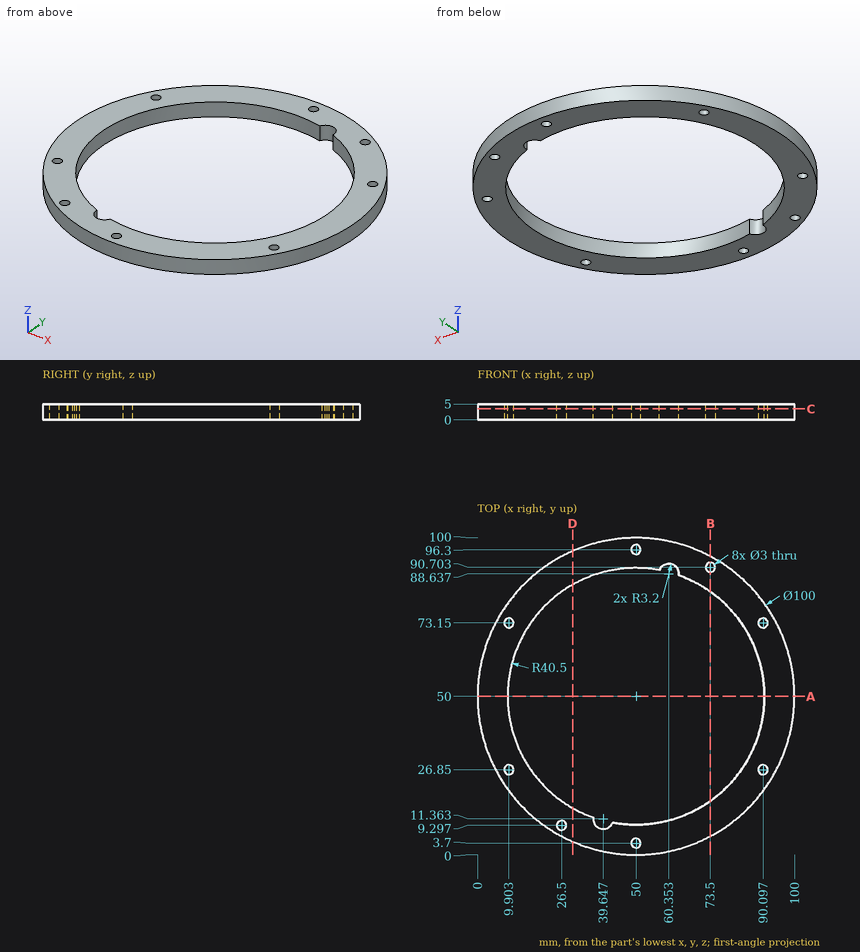
Can you work these out from the drawing? Everything is in mm from the part's minimum corner. Give positions to 0.01 mm unless a question says otherwise; leave off trailing zeros. Order: outer loops, then holes, each group sorted by start corner. A loop starts at its lowest first (then second) coordinate and runs counter-clockwise, first axis right, second up. Notation, with made-up numbers: M -8.5,88.5 L 25.5,88.5 A11 cw 25.5,107.5 Z; hole C 81,82.5 d3. An arc over 180 degrees is marked long. Use a Markdown table: item, result. Add a question column.
Item 1: Suppose I cut it at B-B (x = 73.5). List the corners of the cut face in (y, z) for me (1 decimal).
Item 2: Suppose I cut it at A-A (y = 50). List the corners of the cut face in (x, z) for me, then the cut area to 3 significant figures.
Item 3: If I drill on L1, parallel to Y at x = 50, z = 3.05; L2, parallel to Y at x = 50.5, z = 3.7 (1 decimal); L3, parallel to X at y = 8.5, z = 1.3 (1 decimal), over which ranges is the centre line in solid material (lowest first)? Write a range as [from, to].
Item 4: Suppose I cut it at D-D (x = 30). List the corners of the cut face in (y, z) for me, then the cut area to 3 significant figures.
Item 5: Will these pins go through, and if not, where does the flat tip stop? pin 1 (2.5 mm diameter, centred on x = 50, y = 3.7, fed in from +Z); pin 2 (1.5 mm diameter, centred on x = 23, z = 4.5, fed in from +Y) (1 decimal); pin 3 (1 mm diameter, centred on y = 30.5, z = 3, fed in from +X).
Item 6: Suppose I cut it at C-C (z = 3.5). Count the separate pieces of the cut face and the enclosed holes in it, then the cut area to 3 significant figures.
Answer sheet:
| question | item | result |
|---|---|---|
| 1 | outline | M 5.9,0 L 17,0 L 17,5 L 5.9,5 Z; M 83,0 L 89.2,0 L 89.2,5 L 83,5 Z; M 92.2,0 L 94.1,0 L 94.1,5 L 92.2,5 Z |
| 2 | outline | M 0,0 L 9.5,0 L 9.5,5 L 0,5 Z; M 90.5,0 L 100,0 L 100,5 L 90.5,5 Z |
| 2 | area | 95.0 mm² |
| 3 | L1 | y = [0, 2.2], [5.2, 9.5], [90.5, 94.8], [97.8, 100] |
| 3 | L2 | y = [0, 2.3], [5.1, 9.5], [90.5, 94.9], [97.7, 100] |
| 3 | L3 | x = [22.1, 25.2], [27.8, 38.2], [41.1, 77.9] |
| 4 | outline | M 4.17,0 L 14.78,0 L 14.78,5 L 4.17,5 Z; M 85.22,0 L 95.83,0 L 95.83,5 L 85.22,5 Z |
| 4 | area | 106 mm² |
| 5 | pin 1 | passes through |
| 5 | pin 2 | stops at y = 92.6 |
| 5 | pin 3 | stops at x = 96.25 |
| 6 | separate pieces | 1 |
| 6 | enclosed holes | 9 |
| 6 | area | 2,620 mm² |
